Print and shaded views of the part. All mm, measured from the part's lowest x, y and z. A direction names the side the tool comes from. Give positions to 0.01 mm unless a question says otherwise; leave off trailing zeros. Loops run counter-clockwise (first coordinate to the right, second up) from the corner with the lowest first, then second, coordinate; pieces in that order, holes last. Notation, with made-up numbers: (27, 1) - (77, 1) arc R12 cw to (77, 6) - close; hole circle Ø3 at (12, 44). An arc over 180 degrees is marked (long way). Return JSON: item names as keys, results as strings.
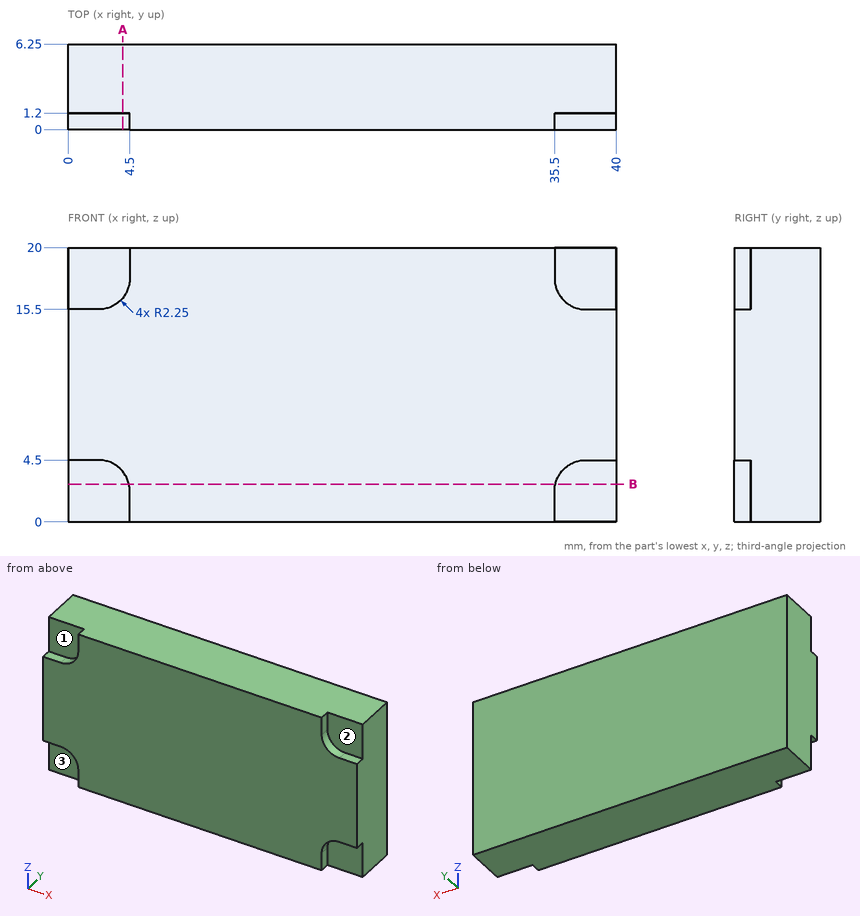
1. Drop flat-ended pins along their axis: P1, Ø2, axis at x = 2.5, z = 2.5, coming from the -Y side; P2, Ø1, axis at y = 0.5, z = 1.5, coming from the -X side; P3, Ø1, axis at y = 0.5, z = 18.5, coming from the +X side. Give the stop position or say it passes through.
Values follow:
{"P1": "stops at y = 1.2", "P2": "stops at x = 4.5", "P3": "stops at x = 35.5"}
2. Cut at A-A, the plane x = 4. Write the cut outline in (y, z), plus the area to 3 significant figures.
Values follow:
{"outline": "(0, 3.66) - (1.2, 3.66) - (1.2, 0) - (6.25, 0) - (6.25, 20) - (1.2, 20) - (1.2, 16.34) - (0, 16.34) - close", "area": "116 mm²"}
3. Cut at B-B, the plane z = 2.75. Write the cut outline in (x, y).
Values follow:
{"outline": "(0, 1.2) - (4.44, 1.2) - (4.44, 0) - (35.56, 0) - (35.56, 1.2) - (40, 1.2) - (40, 6.25) - (0, 6.25) - close"}
4. Which spindle directions (+Z, -Z, +X, -X, +Y, -Y) get a long thin tool onto all of the face, cutting with end or side? Do the marked faces 1, 2 and 3. Say none if no direction does.
Values follow:
{"face 1": "+Z, -X, -Y", "face 2": "+Z, +X, -Y", "face 3": "-Z, -X, -Y"}
